from build123d import *

# Parameters (mm, degrees)
SKETCH1_W           = 25.4
SKETCH1_H           = 25.4
BOSS_EXTRUDE1_DEPTH = 127
CUT_EXTRUDE1_DEPTH  = 127


with BuildPart() as part:
    # Sketch1 → Boss-Extrude1 (new body)
    with BuildSketch(Plane.XY):
        Rectangle(SKETCH1_W, SKETCH1_H)
    extrude(amount=BOSS_EXTRUDE1_DEPTH)

    # 3DSketch1 → Cut-Extrude1 (cut)
    with BuildSketch(Plane(origin=(-9.525, -9.525, 127), x_dir=(0.7071067811865475, 0.7071067811865476, 0), z_dir=(0, 0, -1))):
        Polygon((0, 0), (13.470384182, 13.470384182), (26.940768363, 0), (13.470384182, -13.470384182), align=None)
    extrude(amount=CUT_EXTRUDE1_DEPTH, mode=Mode.SUBTRACT)


solid = part.part
Geometry check sheet. Reference: the model listing, model coordinates, mm. A direction names the side the tool comes from. Round coordinates to 2 decimals unless told otherwise and drop trailing zeros. Loops run counter-clockwise (first coordinate to the right, second up) from the corner with the lowest first, then second, coordinate; pieces in that order, holes last.
Item 1: Gauge pin test, flat end, axial feed: pin 1 (4 mm diameter, centred on x = -7, y = 6.5, fed in from -Z). Record the tip position at first contact, or that the pin passes through.
Item 2: Access from +Z, -Z, +X, -X, +Y, -Y to the whole of each face (thin tool, end or side, straight path). Record for faces 1 (the flat face through (9.525, 0, 64)), 2 (the flat face through (11, 0, 0)).
Item 3: Cross-section at C-C on z = 35. Record the boundary of the cut face in (x, y) (3 decimals).
Item 4: Thickness scan on line 1 (Y direction, x = -3.25, z = 88.5) (3 decimals). Record the ranges inside material, lowest first.
Item 5: Cross-section at A-A on y = -1.5. Record the boundary of the cut face in (x, z) (3 decimals).
Item 6: Mould release check, pull along X, two halves, no side actions. Record for faces 3 (the flat face through (0, -12.7, 63)), 4 (the flat face through (12.7, 0, 63)), 5 (the flat face through (0, 9.525, 64)): pulls with the +X half, pulls with the -X half, needs draft (parallel to the pull), parting line crosses it, or undercut.
Answer sheet:
1. pin 1: passes through
2. face 1: +Z, -Z
2. face 2: -Z, +X, -X, +Y, -Y
3. outline: (-12.7, -12.7) - (12.7, -12.7) - (12.7, 12.7) - (-12.7, 12.7) - close; hole (-9.525, -9.525) - (9.525, -9.525) - (9.525, 9.525) - (-9.525, 9.525) - close
4. line 1: y = -12.7 to -9.525, 9.525 to 12.7
5. outline: (-12.7, 0) - (-9.525, 0) - (-9.525, 127) - (-12.7, 127) - close; (9.525, 0) - (12.7, 0) - (12.7, 127) - (9.525, 127) - close
6. face 3: needs draft
6. face 4: pulls with the +X half
6. face 5: undercut
